Here's the drawing with two shaded views (mm, measured from the low corner). I have some questions. A direction names the side the tool comes from. Coordinates: 2 decimals unless noted, no trailing zeros. Write each loop counter-clockwise with the first axis right and the second up, starting at its lowest first coordinate (ties: lowest second). Pieces come first, ordered by that corner, then holes.
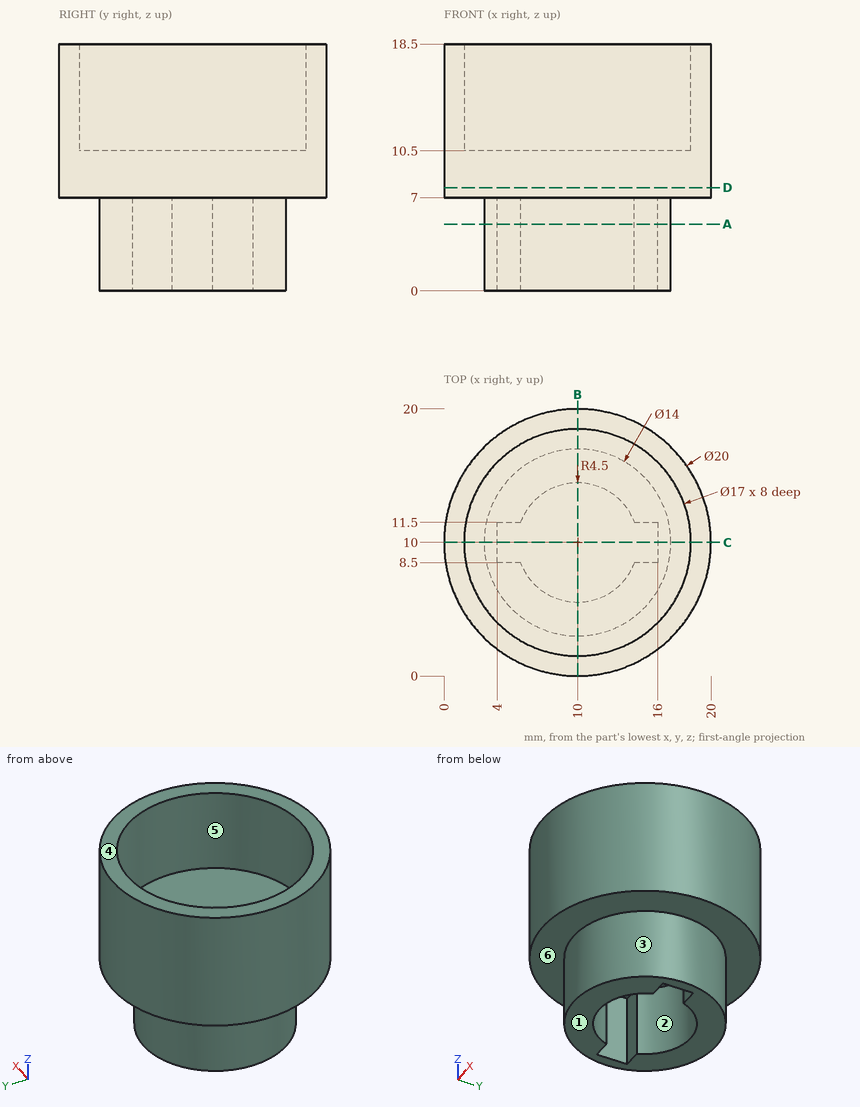
1. Please list where these lines run through material, in increasing order: line 1 along Y through (x, z) = (10, 17.25); line 2 along Z through (x, y) = (11.5, 9); line 3 along Z through (x, y) = (2, 13.5).
Verdict:
line 1: y = 0 to 1.5, 18.5 to 20
line 2: z = 7 to 10.5
line 3: z = 7 to 18.5
2. On a 3-axis mill with a long thin cutter (end or side, diameter ignored), from which of +Z, -Z, +X, -X, +Y, -Y can I reach the whole of each face in a straight line? I mean the marked faces 4, 5 and 6. Say none if no direction works.
Verdict:
face 4: +Z, +X, -X, +Y, -Y
face 5: +Z
face 6: -Z
3. I want a section at A-A on z = 5. Please give me the cut outline in (x, y), plus the area to 3 significant figures.
Verdict:
outline: circle Ø14 at (10, 10); hole (4, 8.5) - (5.76, 8.5) arc R4.5 ccw to (14.24, 8.5) - (16, 8.5) - (16, 11.5) - (14.24, 11.5) arc R4.5 ccw to (5.76, 11.5) - (4, 11.5) - close
area: 80.8 mm2
4. I want a section at B-B on x = 10. Please give me the cut outline in (y, z), plus the area to 3 significant figures.
Verdict:
outline: (0, 7) - (3, 7) - (3, 0) - (5.5, 0) - (5.5, 7) - (14.5, 7) - (14.5, 0) - (17, 0) - (17, 7) - (20, 7) - (20, 18.5) - (18.5, 18.5) - (18.5, 10.5) - (1.5, 10.5) - (1.5, 18.5) - (0, 18.5) - close
area: 129 mm2
5. For pin 1 (8.5 mm diameter, centred on x = 9.5, y = 9, fed in from +Z); pin 2 (3 mm diameter, centred on y = 5.5, z = 2.5, fed in from -X); pin 3 (1.9 mm diameter, centred on x = 4.5, z = 5, fed in from +Y), each with a flat end and sliding along its axis, tell me the tip position at first contact or that it passes through.
Verdict:
pin 1: stops at z = 10.5
pin 2: stops at x = 3.68
pin 3: stops at y = 15.32
6. If we mould it in two halves opening along Y, with no side actions, what happens to the marked faces 1, 2 and 3? For each: pulls with the +Y half, pulls with the -Y half, needs draft (parallel to the pull), parting line crosses it, or undercut.
Verdict:
face 1: needs draft
face 2: undercut
face 3: parting line crosses it
7. I want a section at C-C on y = 10. Please give me the cut outline in (x, z).
Verdict:
outline: (0, 7) - (3, 7) - (3, 0) - (4, 0) - (4, 7) - (16, 7) - (16, 0) - (17, 0) - (17, 7) - (20, 7) - (20, 18.5) - (18.5, 18.5) - (18.5, 10.5) - (1.5, 10.5) - (1.5, 18.5) - (0, 18.5) - close
8. I want a section at D-D on z = 7.75. Please give me the cut outline in (x, y).
Verdict:
outline: circle Ø20 at (10, 10)
